Source: CAD feature listing. Evaluate the final solid. Frame: model axes, mm. Face numbers are marked on the shaded views. A direction names the side the tool comes from. Give positions to 0.01 mm unless a question says otherwise; leave off trailing zeros. Order: outer loops, then holes, each group sorted by start corner. A loop starts at its lowest first (then second) coordinate and runs counter-clockwise, first axis right, second up. Notation, with made-up numbers: (74.5, -10) - (129.5, -10) arc R26 ccw to (129.5, 21) - close; hole circle Ø1 at (-8.5, 40). An arc over 180 degrees is marked (long way). Answer as CSV lines item,"result".
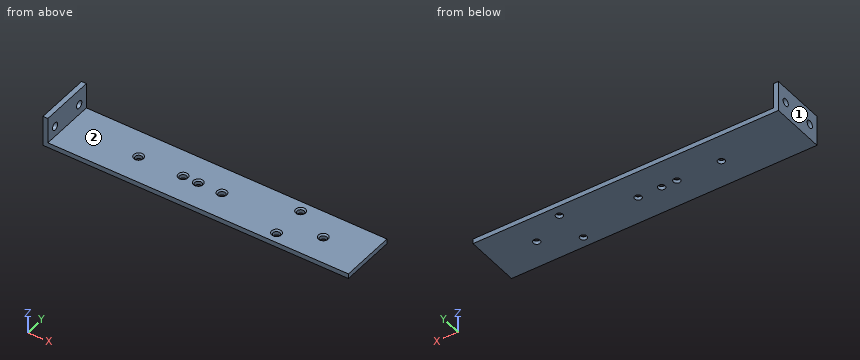
```python
from build123d import *

# Parameters (mm, degrees)
SKETCH_W        = 220
SKETCH_H        = 40
PAD_DEPTH       = 3.5
SKETCH001_R     = 2.5
POCKET_DEPTH    = 3.501
CHAMFER_SIZE    = 1
SKETCH002_W     = 3.5
SKETCH002_H     = 40
PAD001_DEPTH    = 18.5
SKETCH003_R     = 2.75
POCKET001_DEPTH = 220.001


with BuildPart() as part:
    # Sketch → Pad (new body)
    with BuildSketch(Plane.XY):
        with Locations((110, 20)):
            Rectangle(SKETCH_W, SKETCH_H)
    extrude(amount=PAD_DEPTH)

    # Sketch001 (on Face6 of Pad) → Pocket (cut, through all)
    with BuildSketch(Plane.XY.offset(3.5)):
        with Locations((55, 20)):
            Circle(SKETCH001_R)
        with Locations((87, 20)):
            Circle(SKETCH001_R)
        with Locations((98, 20)):
            Circle(SKETCH001_R)
        with Locations((115, 20)):
            Circle(SKETCH001_R)
        with Locations((188, 20)):
            Circle(SKETCH001_R)
        with Locations((163, 32.5)):
            Circle(SKETCH001_R)
        with Locations((163, 7.5)):
            Circle(SKETCH001_R)
    extrude(amount=-POCKET_DEPTH, mode=Mode.SUBTRACT)

    # Chamfer
    chamfer_edges = [part.edges().sort_by_distance(p)[0] for p in [
        (52.5, 20, 3.5),
        (84.5, 20, 3.5),
        (95.5, 20, 3.5),
        (112.5, 20, 3.5),
        (160.5, 32.5, 3.5),
        (160.5, 7.5, 3.5),
        (185.5, 20, 3.5),
    ]]
    chamfer(chamfer_edges, length=CHAMFER_SIZE)

    # Sketch002 (on Face1 of Chamfer) → Pad001 (join)
    with BuildSketch(Plane.XY.offset(3.5)):
        with Locations((1.75, 20)):
            Rectangle(SKETCH002_W, SKETCH002_H)
    extrude(amount=PAD001_DEPTH)

    # Sketch003 → Pocket001 (cut, through all)
    with BuildSketch(Plane(origin=(0, 0, 0), x_dir=(0, -1, 0), z_dir=(-1, 0, 0))):
        with Locations((-32.5, 11)):
            Circle(SKETCH003_R)
        with Locations((-7.5, 11)):
            Circle(SKETCH003_R)
    extrude(amount=-POCKET001_DEPTH, mode=Mode.SUBTRACT)


solid = part.part
```
(1) Cut plane B-B (y = 7.5). Return loops of the section in (x, z), then the cut area to 3 significant figures.
Completed:
outline,"(0, 0) - (160.5, 0) - (160.5, 2.5) - (159.5, 3.5) - (3.5, 3.5) - (3.5, 8.25) - (0, 8.25) - close; (0, 13.75) - (3.5, 13.75) - (3.5, 22) - (0, 22) - close; (165.5, 0) - (220, 0) - (220, 3.5) - (166.5, 3.5) - (165.5, 2.5) - close"
area,"797 mm²"
(2) Ray query, line 1 (Y direction, x = 87, z = 0.8); line 2 (Z direction, x = 133.5, y = 11.5). Return the intervals inside material, ascending. Write a range as from..to.
Completed:
line 1,"0..17.5, 22.5..40"
line 2,"0..3.5"
(3) Cut plane A-A (x = 115). Return loops of the section in (y, z).
Completed:
outline,"(0, 0) - (17.5, 0) - (17.5, 2.5) - (16.5, 3.5) - (0, 3.5) - close; (22.5, 0) - (40, 0) - (40, 3.5) - (23.5, 3.5) - (22.5, 2.5) - close"
(4) Cut plane D-D (z = 17.75). Return loops of the section in (x, y), then the cut area to 3 significant figures.
Completed:
outline,"(0, 0) - (3.5, 0) - (3.5, 40) - (0, 40) - close"
area,"140 mm²"
(5) Cut plane C-C (y = 25.5). Return loops of the section in (x, z).
Completed:
outline,"(0, 0) - (220, 0) - (220, 3.5) - (3.5, 3.5) - (3.5, 22) - (0, 22) - close"
(6) Contact query for flat-ended pins moving along their axis: pin 1 (6.5 mm diameter, centred on x = 188, y = 20, fed in from +Z); pin 2 (4.5 mm diameter, centred on x = 115, y = 20, fed in from -Z); pin 3 (2 mm diameter, centred on y = 7.5, z = 17, fed in from -X); pin 4 (12 mm diameter, centred on x = 32, y = 23, fed in from +Z). Output: stop coordinate, or through.
Completed:
pin 1,"z = 3.25"
pin 2,"through"
pin 3,"x = 0"
pin 4,"z = 3.5"
(7) Access query for the marked faces 1 and 2. Directions: +Z, -Z, +X, -X, +Y, -Y. A direction counts if a zero-diameter tool reaches every point of the face in a straight line with its end or side. Return the directions, or none.
Completed:
face 1,"+Z, -Z, -X, +Y, -Y"
face 2,"+Z, +X, +Y, -Y"
